```python
from build123d import *

# Parameters (mm, degrees)
F1_DEPTH      = 1132
F2_W          = 143
F2_H          = 4
F3_DEPTH      = 8.001
F3_DEPTH_BACK = 4.001


with BuildPart() as f1:
    # F0 (on Front) → F1 (new body)
    with BuildSketch(Plane.XZ):
        Polygon((95.6217723169, 0), (0, 0), (1.6568542495, -4), (95.971726971, -4), (118.6568542495, 0), (238.971726971, 0), (261.6568542495, 4), (311.6568542495, 4), (311.6568542495, 8), (261.3068995954, 8), (238.6217723169, 4), (118.3068995954, 4), align=None)
    extrude(amount=-F1_DEPTH)

    # F2 (on face) → F3 (cut, two sides)
    with BuildSketch(Plane.XY.offset(4)) as f3_sk:
        with Locations((240.1568542495, 191)):
            Rectangle(F2_W, F2_H)
        with Locations((240.1568542495, 441)):
            Rectangle(F2_W, F2_H)
        with Locations((240.1568542495, 691)):
            Rectangle(F2_W, F2_H)
        with Locations((240.1568542495, 941)):
            Rectangle(F2_W, F2_H)
    extrude(amount=-F3_DEPTH, mode=Mode.SUBTRACT)
    extrude(f3_sk.sketch, amount=F3_DEPTH_BACK, mode=Mode.SUBTRACT)


solid = f1.part
```
Verification items for the finished model (mm, model axes). A direction names the side the tool comes from. Coordinates: 2 decimals unless noted, no trailing zeros. Loops run counter-clockwise (first coordinate to the right, second up) from the corner with the lowest first, then second, coordinate; pieces in that order, holes last. Notation, with made-up numbers: (45, 32) -> (88, 32) arc R12 cw to (88, 46) -> close; hole circle Ø5 at (72, 27.5). An arc over 180 degrees is marked (long way). Answer in a Markdown table with one row per item. Add a question column.
1. Access from +Z, -Z, +X, -X, +Y, -Y to the whole of each face (thin tool, end or side, straight path). Record for faces 1 (the face through (286, 564, 4)), 2 (the face through (287, 93, 8)), 3 (the face through (179, 558, 4)).
2. Section check B-B, the plane y = 227.5. Enter the section's corners in (x, z).
3. Depth check by flat-ended pin: P1, Ø1.2, axis at y = 690, z = 2.5, coming from the +X side; P2, Ø10, axis at x = 125.5, y = 600.5, coming from the -Z side; P3, Ø15, axis at x = 289, y = 871, coming from the -Z side. Enter the tip coordinate at first touch or a pass-through.
4. Section check A-A, the plane x = 206.5. Enter the section's corners in (y, z).
5. Material ranges on probe 1 along Y at (x, z) = (209.5, 1); probe 2 along Z at (x, y) = (221, 1018.5); probe 3 along Z at (x, y) = (93, 429.5), recorded low to high. Write a range as [from, to].
Derived:
| question | item | result |
|---|---|---|
| 1 | face 1 | -Z, +X, +Y, -Y |
| 1 | face 2 | +Z, +X, -X, +Y, -Y |
| 1 | face 3 | +Z, -X, +Y, -Y |
| 2 | outline | (0, 0) -> (1.66, -4) -> (95.97, -4) -> (118.66, 0) -> (238.97, 0) -> (261.66, 4) -> (311.66, 4) -> (311.66, 8) -> (261.31, 8) -> (238.62, 4) -> (118.31, 4) -> (95.62, 0) -> close |
| 3 | P1 | stops at x = 168.66 |
| 3 | P2 | stops at z = 0 |
| 3 | P3 | stops at z = 4 |
| 4 | outline | (0, 0) -> (189, 0) -> (189, 4) -> (0, 4) -> close; (193, 0) -> (439, 0) -> (439, 4) -> (193, 4) -> close; (443, 0) -> (689, 0) -> (689, 4) -> (443, 4) -> close; (693, 0) -> (939, 0) -> (939, 4) -> (693, 4) -> close; (943, 0) -> (1132, 0) -> (1132, 4) -> (943, 4) -> close |
| 5 | probe 1 | y = [0, 189], [193, 439], [443, 689], [693, 939], [943, 1132] |
| 5 | probe 2 | z = [0, 4] |
| 5 | probe 3 | z = [-4, 0] |
